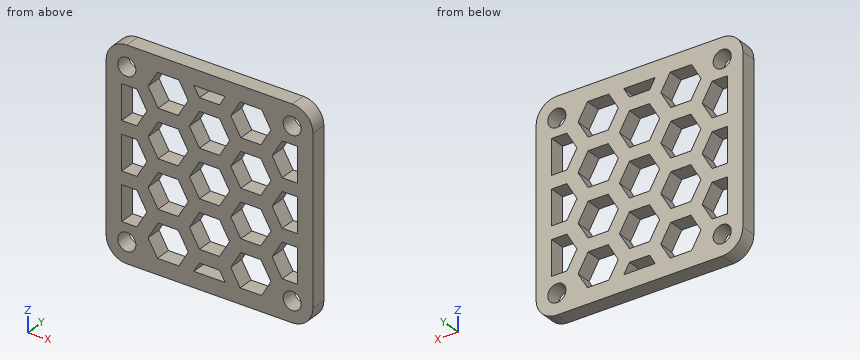
```python
from build123d import *

# Parameters (mm, degrees)
SKETCH1_R           = 1.75
BOSS_EXTRUDE1_DEPTH = 3
CUT_EXTRUDE1_DEPTH  = 29.442925307
BOSS_EXTRUDE2_DEPTH = 3
SKETCH1_3_R         = 1.75
CUT_EXTRUDE2_DEPTH  = 29.442925307


with BuildPart() as part:
    # Sketch1 → Boss-Extrude1 (new body)
    # profile 1 of 5: a face of its own
    with BuildSketch(Plane(origin=(0, 0, 0), x_dir=(1, 0, 0), z_dir=(0, 1, 0))):
        with BuildLine():
            Line((-16, -20), (16, -20))
            ThreePointArc((16, -20), (18.828427125, -18.828427125), (20, -16))
            Line((20, -16), (20, 16))
            ThreePointArc((20, 16), (18.828427125, 18.828427125), (16, 20))
            Line((16, 20), (-16, 20))
            ThreePointArc((-16, 20), (-18.828427125, 18.828427125), (-20, 16))
            Line((-20, 16), (-20, -16))
            ThreePointArc((-20, -16), (-18.828427125, -18.828427125), (-16, -20))
        make_face()
        with Locations((-16, 16)):
            Circle(SKETCH1_R, mode=Mode.SUBTRACT)
        with Locations((16, 16)):
            Circle(SKETCH1_R, mode=Mode.SUBTRACT)
        with Locations((16, -16)):
            Circle(SKETCH1_R, mode=Mode.SUBTRACT)
        with Locations((-16, -16)):
            Circle(SKETCH1_R, mode=Mode.SUBTRACT)
    # profile 2 of 5: a face of its own
    with BuildSketch(Plane(origin=(0, 0, 0), x_dir=(1, 0, 0), z_dir=(0, 1, 0))):
        with Locations((-16, 16)):
            Circle(SKETCH1_R)
    # profile 3 of 5: a face of its own
    with BuildSketch(Plane(origin=(0, 0, 0), x_dir=(1, 0, 0), z_dir=(0, 1, 0))):
        with Locations((16, 16)):
            Circle(SKETCH1_R)
    # profile 4 of 5: a face of its own
    with BuildSketch(Plane(origin=(0, 0, 0), x_dir=(1, 0, 0), z_dir=(0, 1, 0))):
        with Locations((16, -16)):
            Circle(SKETCH1_R)
    # profile 5 of 5: a face of its own
    with BuildSketch(Plane(origin=(0, 0, 0), x_dir=(1, 0, 0), z_dir=(0, 1, 0))):
        with Locations((-16, -16)):
            Circle(SKETCH1_R)
    extrude(amount=BOSS_EXTRUDE1_DEPTH)

    # Sketch3 → Cut-Extrude1 (cut, through all)
    with BuildSketch(Plane(origin=(0, 0, 0), x_dir=(1, 0, 0), z_dir=(0, 1, 0))):
        Polygon((6.05502117, -1.25), (4.11004234, -4.618802154), (6.05502117, -7.987604307), (9.94497883, -7.987604307), (11.88995766, -4.618802154), (9.94497883, -1.25), align=None)
        Polygon((-1.94497883, 3.368802154), (-3.88995766, 0), (-1.94497883, -3.368802154), (1.94497883, -3.368802154), (3.88995766, 0), (1.94497883, 3.368802154), align=None)
        Polygon((14.05502117, 3.368802154), (12.11004234, 0), (14.05502117, -3.368802154), (17.94497883, -3.368802154), (19.88995766, 0), (17.94497883, 3.368802154), align=None)
        Polygon((22.05502117, -1.25), (20.11004234, -4.618802154), (22.05502117, -7.987604307), (25.94497883, -7.987604307), (27.88995766, -4.618802154), (25.94497883, -1.25), align=None)
        Polygon((14.05502117, 12.606402154), (12.11004234, 9.2376), (14.05502117, 5.868797846), (17.94497883, 5.868797846), (19.88995766, 9.2376), (17.94497883, 12.606402154), align=None)
        Polygon((22.05502117, 7.9876), (20.11004234, 4.618797846), (22.05502117, 1.249995693), (25.94497883, 1.249995693), (27.88995766, 4.618797846), (25.94497883, 7.9876), align=None)
        Polygon((14.05502117, 21.844002154), (12.11004234, 18.4752), (14.05502117, 15.106397846), (17.94497883, 15.106397846), (19.88995766, 18.4752), (17.94497883, 21.844002154), align=None)
        Polygon((22.05502117, 17.2252), (20.11004234, 13.856397846), (22.05502117, 10.487595693), (25.94497883, 10.487595693), (27.88995766, 13.856397846), (25.94497883, 17.2252), align=None)
        Polygon((-1.94497883, 12.606402154), (-3.88995766, 9.2376), (-1.94497883, 5.868797846), (1.94497883, 5.868797846), (3.88995766, 9.2376), (1.94497883, 12.606402154), align=None)
        Polygon((6.05502117, 7.9876), (4.11004234, 4.618797846), (6.05502117, 1.249995693), (9.94497883, 1.249995693), (11.88995766, 4.618797846), (9.94497883, 7.9876), align=None)
        Polygon((-1.94497883, 21.844002154), (-3.88995766, 18.4752), (-1.94497883, 15.106397846), (1.94497883, 15.106397846), (3.88995766, 18.4752), (1.94497883, 21.844002154), align=None)
        Polygon((6.05502117, 17.2252), (4.11004234, 13.856397846), (6.05502117, 10.487595693), (9.94497883, 10.487595693), (11.88995766, 13.856397846), (9.94497883, 17.2252), align=None)
        Polygon((-9.94497883, -1.25), (-6.05502117, -1.25), (-4.11004234, -4.618802154), (-6.05502117, -7.987604307), (-9.94497883, -7.987604307), (-11.88995766, -4.618802154), align=None)
        Polygon((-9.94497883, 7.9876), (-6.05502117, 7.9876), (-4.11004234, 4.618797846), (-6.05502117, 1.249995693), (-9.94497883, 1.249995693), (-11.88995766, 4.618797846), align=None)
        Polygon((-9.94497883, 17.2252), (-6.05502117, 17.2252), (-4.11004234, 13.856397846), (-6.05502117, 10.487595693), (-9.94497883, 10.487595693), (-11.88995766, 13.856397846), align=None)
        Polygon((-17.94497883, 12.606402154), (-14.05502117, 12.606402154), (-12.11004234, 9.2376), (-14.05502117, 5.868797846), (-17.94497883, 5.868797846), (-19.88995766, 9.2376), align=None)
        Polygon((-17.94497883, 3.368802154), (-14.05502117, 3.368802154), (-12.11004234, 0), (-14.05502117, -3.368802154), (-17.94497883, -3.368802154), (-19.88995766, 0), align=None)
        Polygon((-25.94497883, -1.25), (-22.05502117, -1.25), (-20.11004234, -4.618802154), (-22.05502117, -7.987604307), (-25.94497883, -7.987604307), (-27.88995766, -4.618802154), align=None)
        Polygon((-25.94497883, 7.9876), (-22.05502117, 7.9876), (-20.11004234, 4.618797846), (-22.05502117, 1.249995693), (-25.94497883, 1.249995693), (-27.88995766, 4.618797846), align=None)
        Polygon((-25.94497883, 17.2252), (-22.05502117, 17.2252), (-20.11004234, 13.856397846), (-22.05502117, 10.487595693), (-25.94497883, 10.487595693), (-27.88995766, 13.856397846), align=None)
        Polygon((-17.94497883, 21.844002154), (-14.05502117, 21.844002154), (-12.11004234, 18.4752), (-14.05502117, 15.106397846), (-17.94497883, 15.106397846), (-19.88995766, 18.4752), align=None)
        Polygon((17.94497883, -21.844002154), (14.05502117, -21.844002154), (12.11004234, -18.4752), (14.05502117, -15.106397846), (17.94497883, -15.106397846), (19.88995766, -18.4752), align=None)
        Polygon((25.94497883, -17.2252), (22.05502117, -17.2252), (20.11004234, -13.856397846), (22.05502117, -10.487595693), (25.94497883, -10.487595693), (27.88995766, -13.856397846), align=None)
        Polygon((17.94497883, -12.606402154), (14.05502117, -12.606402154), (12.11004234, -9.2376), (14.05502117, -5.868797846), (17.94497883, -5.868797846), (19.88995766, -9.2376), align=None)
        Polygon((9.94497883, -17.2252), (6.05502117, -17.2252), (4.11004234, -13.856397846), (6.05502117, -10.487595693), (9.94497883, -10.487595693), (11.88995766, -13.856397846), align=None)
        Polygon((1.94497883, -21.844002154), (-1.94497883, -21.844002154), (-3.88995766, -18.4752), (-1.94497883, -15.106397846), (1.94497883, -15.106397846), (3.88995766, -18.4752), align=None)
        Polygon((1.94497883, -12.606402154), (-1.94497883, -12.606402154), (-3.88995766, -9.2376), (-1.94497883, -5.868797846), (1.94497883, -5.868797846), (3.88995766, -9.2376), align=None)
        Polygon((-11.88995766, -13.856397846), (-9.94497883, -17.2252), (-6.05502117, -17.2252), (-4.11004234, -13.856397846), (-6.05502117, -10.487595693), (-9.94497883, -10.487595693), align=None)
        Polygon((-19.88995766, -18.4752), (-17.94497883, -21.844002154), (-14.05502117, -21.844002154), (-12.11004234, -18.4752), (-14.05502117, -15.106397846), (-17.94497883, -15.106397846), align=None)
        Polygon((-27.88995766, -13.856397846), (-25.94497883, -17.2252), (-22.05502117, -17.2252), (-20.11004234, -13.856397846), (-22.05502117, -10.487595693), (-25.94497883, -10.487595693), align=None)
        Polygon((-19.88995766, -9.2376), (-17.94497883, -12.606402154), (-14.05502117, -12.606402154), (-12.11004234, -9.2376), (-14.05502117, -5.868797846), (-17.94497883, -5.868797846), align=None)
    extrude(amount=CUT_EXTRUDE1_DEPTH, mode=Mode.SUBTRACT)

    # Sketch4 → Boss-Extrude2 (add, through all)
    with BuildSketch(Plane(origin=(0, 0, 0), x_dir=(1, 0, 0), z_dir=(0, 1, 0))):
        with BuildLine():
            Line((-20, 16), (-20, -16))
            ThreePointArc((-20, -16), (-18.828427125, -18.828427125), (-16, -20))
            Line((-16, -20), (16, -20))
            ThreePointArc((16, -20), (18.828427125, -18.828427125), (20, -16))
            Line((20, -16), (20, 16))
            ThreePointArc((20, 16), (18.828427125, 18.828427125), (16, 20))
            Line((16, 20), (-16, 20))
            ThreePointArc((-16, 20), (-18.828427125, 18.828427125), (-20, 16))
        make_face()
        Polygon((12.961749457, 17), (-12.961749457, 17), (-14.05502117, 15.106397846), (-17, 15.106397846), (-17, -15.106397846), (-14.05502117, -15.106397846), (-12.961749457, -17), (12.961749457, -17), (14.05502117, -15.106397846), (17, -15.106397846), (17, 15.106397846), (14.05502117, 15.106397846), align=None, mode=Mode.SUBTRACT)
    extrude(amount=BOSS_EXTRUDE2_DEPTH)

    # Sketch1<3> → Cut-Extrude2 (cut, through all)
    with BuildSketch(Plane(origin=(0, 0, 0), x_dir=(1, 0, 0), z_dir=(0, 1, 0))):
        with Locations(Location((16, 16, 0), (0, 0, 270))):
            Circle(SKETCH1_3_R)
        with Locations(Location((-16, -16, 0), (0, 0, 270))):
            Circle(SKETCH1_3_R)
        with Locations(Location((16, -16, 0), (0, 0, 270))):
            Circle(SKETCH1_3_R)
        with Locations(Location((-16, 16, 0), (0, 0, 270))):
            Circle(SKETCH1_3_R)
    extrude(amount=CUT_EXTRUDE2_DEPTH, mode=Mode.SUBTRACT)


solid = part.part
```
For this review, take the finished solid that the model builds, in its own axes (mm). Give positions to 0.01 mm unless a question says otherwise; leave off trailing zeros. Write each loop counter-clockwise with the first axis right and the second up, starting at its lowest first coordinate (ties: lowest second). Pieces come first, ordered by that corner, then holes. Notation, with made-up numbers: M -38.75,75.25 L -28.75,75.25 A27 cw -28.75,103.25 Z; hole C 23,9 d3. An arc over 180 degrees is marked long. Answer as a JSON object with one key per item and string values. Group by question number.
Item 1: Consider section C-C on y = 0.7. Count the separate pieces of the cut face and the enclosed holes in it, plus the area to 3 significant figures.
Item 2: For probe 1 along Z at (x, y) = (16, 2.35); probe 2 along Z at (x, y) = (-9, 2.5); probe 3 along Z at (x, y) = (5, 0.75), list the stretches that pass through material, from the lowest coordinate up. Write a range as [from, to].
Item 3: Consider section D-D on z = 16.5. Write out the cut boundary in (x, y).
Item 4: For pin 1 Ø4 at (x, z) = (10, 5) entering from -Y, flat-tipped, find the tip position at first contact; note if it passes through.
Item 5: Consider section A-A on x = 0. Write out the cut boundary in (y, z).
Item 6: Consider section B-B on z = 8.5. Write out the cut boundary in (x, y), plus the area to 3 significant figures.
Check result:
{
 "1": {"separate pieces": "1", "enclosed holes": "23", "area": "942 mm^2"},
 "2": {"probe 1": "z = [-20, -17.75], [-14.25, -12.61], [-5.87, -3.37], [3.37, 5.87], [12.61, 14.25], [17.75, 20]", "probe 2": "z = [-20, -17], [-10.49, -7.99], [-1.25, 1.25], [7.99, 10.49], [17, 20]", "probe 3": "z = [-20, -15.4], [-12.31, -6.16], [-3.08, 3.08], [6.16, 12.31], [15.4, 20]"},
 "3": {"outline": "M -19.97,0 L -17.68,0 L -17.68,3 L -19.97,3 Z; M -14.32,0 L -10.36,0 L -10.36,3 L -14.32,3 Z; M -5.64,0 L -2.75,0 L -2.75,3 L -5.64,3 Z; M 2.75,0 L 5.64,0 L 5.64,3 L 2.75,3 Z; M 10.36,0 L 14.32,0 L 14.32,3 L 10.36,3 Z; M 17.68,0 L 19.97,0 L 19.97,3 L 17.68,3 Z"},
 "4": {"pin 1": "stops at y = 0"},
 "5": {"outline": "M 0,-20 L 3,-20 L 3,-17 L 0,-17 Z; M 0,-15.11 L 3,-15.11 L 3,-12.61 L 0,-12.61 Z; M 0,-5.87 L 3,-5.87 L 3,-3.37 L 0,-3.37 Z; M 0,3.37 L 3,3.37 L 3,5.87 L 0,5.87 Z; M 0,12.61 L 3,12.61 L 3,15.11 L 0,15.11 Z; M 0,17 L 3,17 L 3,20 L 0,20 Z"},
 "6": {"outline": "M -20,0 L -17,0 L -17,3 L -20,3 Z; M -12.54,0 L -3.46,0 L -3.46,3 L -12.54,3 Z; M 3.46,0 L 12.54,0 L 12.54,3 L 3.46,3 Z; M 17,0 L 20,0 L 20,3 L 17,3 Z", "area": "72.4 mm^2"}
}
